from build123d import *

# Parameters (mm, degrees)
F3_DEPTH  = 12.7
F4_R      = 1.27
F5_DEPTH  = 2.54
F6_R      = 1.27
F7_DEPTH  = 2.54
F5_FACE_R = 1.27
F8_DEPTH  = 5.08
F7_FACE_R = 1.27
F9_DEPTH  = 5.08
F10_R     = 3.342625
F11_DEPTH = 42.164


with BuildPart() as f1:
    # F0 (on Front) → F1 (revolve)
    with BuildSketch(Plane.XZ):
        with BuildLine():
            ThreePointArc((0, -29.039641), (20.534127, -20.534127), (29.039641, 0))
            ThreePointArc((29.039641, 0), (20.534127, 20.534127), (0, 29.039641))
            Line((0, 29.039641), (0, -29.039641))
        make_face()
    revolve(axis=Axis((0, 0, 0), (0, 0, -1)))

    # F2 (on Right) → F3 (cut, symmetric)
    with BuildSketch(Plane.YZ):
        Polygon((-32.992329, 28.453402), (0, 28.453402), (29.31824, 28.453402), (29.31824, 34.250099), (-32.992329, 34.250099), align=None)
        Polygon((29.438438, -28.448), (-32.842074, -28.448), (-32.842074, -37.691581), (29.31824, -37.691581), (29.31824, -29.660275), align=None)
    extrude(amount=F3_DEPTH, both=True, mode=Mode.SUBTRACT)

    # F4 (on face) → F5 (cut)
    with BuildSketch(Plane(origin=(0, 0, -28.448), x_dir=(1, 0, 0), z_dir=(0, 0, -1))):
        Circle(F4_R)
    extrude(amount=-F5_DEPTH, mode=Mode.SUBTRACT)

    # F6 (on face) → F7 (cut)
    with BuildSketch(Plane.XY.offset(28.453402)):
        Circle(F6_R)
    extrude(amount=-F7_DEPTH, mode=Mode.SUBTRACT)

    # F5_face (on face) → F8 (join)
    with BuildSketch(Plane(origin=(0, 0, -25.908), x_dir=(1, 0, 0), z_dir=(0, 0, -1))):
        Circle(F5_FACE_R)
    extrude(amount=F8_DEPTH)

    # F7_face (on face) → F9 (join)
    with BuildSketch(Plane.XY.offset(25.913402)):
        Circle(F7_FACE_R)
    extrude(amount=F9_DEPTH)

    # F10 (on Front) → F11 (cut, symmetric)
    with BuildSketch(Plane.XZ):
        Circle(F10_R)
    extrude(amount=F11_DEPTH, both=True, mode=Mode.SUBTRACT)


solid = f1.part
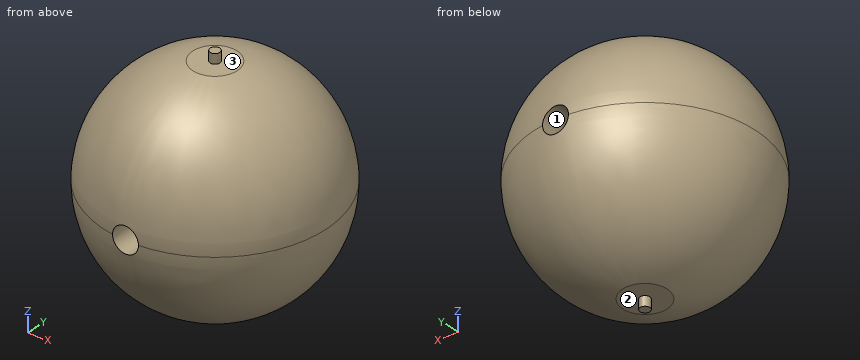
Geometry check sheet. Reference: the model listing, model coordinates, mm. Face numbers are marked on the shaded views. Give positions to 0.01 mm unless a question says otherwise; leave off trailing zeros. Put each result on its own line as item: value.
1. Draft check along Z on the marked faces 1, 2 and 3. Enter one of: +Z half, -Z half, draft (parallel to the pull), parting line (faces both ways), or undercut.
Ans:
face 1: undercut
face 2: -Z half
face 3: +Z half
2. Thickness scan on line 1 (Z direction, x = 0, y = 3); line 2 (Z direction, x = -0.5, y = -9); line 3 (Y direction, x = 23.5, z = 7). Record the ranges inside material, lowest first.
Ans:
line 1: z = -28.45 to -3.34, 3.34 to 28.45
line 2: z = -27.61 to -3.31, 3.31 to 27.61
line 3: y = -15.56 to 15.56
3. Go/stop test with flat-tipped pins: pin 1 (6 mm diameter, centred on y = -13, z = 2.5, fed in from +X) (3 decimals); pin 2 (1.5 mm diameter, centred on y = 2, z = 14.5, fed in from +X); pin 3 (4 mm diameter, centred on y = 12, z = -13, fed in from +X) (3 decimals); pin 4 (13 mm diameter, centred on x = 2, y = -1.5, fed in from +Z). Record where each tip stops, or that it passes through.
Ans:
pin 1: stops at x = 27.175
pin 2: stops at x = 25.5
pin 3: stops at x = 24.435
pin 4: stops at z = 30.99
